Here's how the part is built. I have some questions about the finished solid (model axes, mm). A direction names the side the tool comes from. Round coordinates to 2 decimals unless told otherwise and drop trailing zeros. Loops run counter-clockwise (first coordinate to the right, second up) from the corner with the lowest first, then second, coordinate; pieces in that order, holes last. Notation, with made-up numbers: M -34,-11.5 L 20,-11.5 A9 ccw 20,-5.5 Z; hole C 73.5,19.5 d11. An arc over 180 degrees is marked long. Answer as a JSON object with one key per item and string values.
from build123d import *

# Parameters (mm, degrees)
SKETCH002_W     = 16
SKETCH002_H     = 25.5
PAD_DEPTH       = 1.5
SKETCH003_R     = 2.25
PAD001_DEPTH    = 2.9
SKETCH004_R     = 2.25
PAD002_DEPTH    = 2.9
POCKET_DEPTH    = 11.35
POCKET001_DEPTH = 11.35
FILLET_R        = 1.2


with BuildPart() as part:
    # Sketch002 → Pad (new body)
    with BuildSketch(Plane.XY):
        Rectangle(SKETCH002_W, SKETCH002_H)
        with BuildLine():
            ThreePointArc((1, 4.75), (2.5, 3.25), (4, 4.75))
            Line((4, 4.75), (4, 5.25))
            ThreePointArc((4, 5.25), (2.5, 6.75), (1, 5.25))
            Line((1, 4.75), (1, 5.25))
        make_face(mode=Mode.SUBTRACT)
        with BuildLine():
            ThreePointArc((-1, -4.75), (-2.5, -3.25), (-4, -4.75))
            Line((-4, -4.75), (-4, -5.25))
            ThreePointArc((-4, -5.25), (-2.5, -6.75), (-1, -5.25))
            Line((-1, -4.75), (-1, -5.25))
        make_face(mode=Mode.SUBTRACT)
    extrude(amount=PAD_DEPTH)

    # Sketch003 → Pad001 (join)
    with BuildSketch(Plane.XZ.offset(12.75)):
        with BuildLine():
            ThreePointArc((12.25, 0), (18.500032, 6.25), (12.25, 12.5))
            Line((12.25, 12.5), (0.660254, 12.5))
            Line((0.660254, 12.5), (-8, 7.5))
            Line((-8, 7.5), (-8, 0))
            Line((-8, 0), (12.25, 0))
        make_face()
        with Locations((12.25, 6.25)):
            Circle(SKETCH003_R, mode=Mode.SUBTRACT)
    extrude(amount=-PAD001_DEPTH)

    # Sketch004 → Pad002 (join)
    with BuildSketch(Plane.XZ.offset(-12.75)):
        with BuildLine():
            Line((12.25, 0), (-8, 0))
            Line((-8, 0), (-8, 7.5))
            Line((-8, 7.5), (0.660254, 12.5))
            Line((0.660254, 12.5), (12.25, 12.5))
            ThreePointArc((12.25, 0), (18.500035, 6.25), (12.25, 12.5))
        make_face()
        with Locations((12.250035, 6.25)):
            Circle(SKETCH004_R, mode=Mode.SUBTRACT)
    extrude(amount=PAD002_DEPTH)

    # Sketch005 → Pocket (cut)
    with BuildSketch(Plane.XZ.offset(11.35)):
        with BuildLine():
            Line((18.6, 12.5), (18.6, 0))
            Line((8, 0), (18.6, 0))
            Line((8, 1.005956), (8, 0))
            ThreePointArc((6.50892, 9.8), (5.594985, 5.121605), (8, 1.005956))
            Line((6.50892, 9.8), (11.5, 9.8))
            Line((11.5, 9.8), (11.5, 12.5))
            Line((11.5, 12.5), (18.6, 12.5))
        make_face()
    extrude(amount=-POCKET_DEPTH, mode=Mode.SUBTRACT)

    # Sketch006 → Pocket001 (cut)
    with BuildSketch(Plane.XZ.offset(-11.35)):
        with BuildLine():
            Line((18.6, 12.5), (18.6, 0))
            Line((8, 0), (18.6, 0))
            Line((8, 1.005956), (8, 0))
            ThreePointArc((6.50892, 9.8), (5.594985, 5.121605), (8, 1.005956))
            Line((6.50892, 9.8), (11.5, 9.8))
            Line((11.5, 9.8), (11.5, 12.5))
            Line((11.5, 12.5), (18.6, 12.5))
        make_face()
    extrude(amount=POCKET001_DEPTH, mode=Mode.SUBTRACT)

    # Fillet
    fillet_edges = [part.edges().sort_by_distance(p)[0] for p in [
        (-0.272916, 9.85, 1.5),
        (-0.272916, -9.85, 1.5),
    ]]
    fillet(fillet_edges, radius=FILLET_R)


solid = part.part
Item 1: I want a section at C-C on y = 10.5. List the corners of the cut face in (x, z) for me, plus the area to 3 significant figures.
Solution:
{"outline": "M -8,0 L 8,0 L 8,1.01 A6.75 cw 6.51,9.8 L 11.5,9.8 L 11.5,12.5 L 0.66,12.5 L -8,7.5 Z", "area": "171 mm2"}
Item 2: We'd pull the mould along Y, two halves only. Please class faces 6 (the face through (5, 12.75, 6)), 7 (the face through (10, -12.1, 6.3)), 8 (the face through (2.47, 3.25, 0.74)): +Y half, -Y half, draft (parallel to the pull), parting line (faces both ways), or undercut.
Solution:
{"face 6": "+Y half", "face 7": "draft", "face 8": "undercut"}
Item 3: If I drill on L1, parallel to Y at x = 13, z = 9; L2, parallel to Y at x = -6, z = 8.25; L3, parallel to Z at x = 12.25, y = -11.65, over which ranges is the centre line in solid material (lowest first)? Write a range as from..to.
Solution:
{"L1": "y = -12.75..-11.35, 11.35..12.75", "L2": "y = -12.75..-9.85, 9.85..12.75", "L3": "z = 0..4, 8.5..12.5"}
Item 4: I want a section at D-D on x = 13.25. List the corners of the cut face in (y, z) for me.
Solution:
{"outline": "M -12.75,0.08 L -11.35,0.08 L -11.35,4.23 L -12.75,4.23 Z; M -12.75,8.27 L -11.35,8.27 L -11.35,12.42 L -12.75,12.42 Z; M 11.35,0.08 L 12.75,0.08 L 12.75,4.23 L 11.35,4.23 Z; M 11.35,8.27 L 12.75,8.27 L 12.75,12.42 L 11.35,12.42 Z"}
Item 5: I want a section at A-A on x = 2.5. List the corners of the cut face in (y, z) for me, plus the area to 3 significant figures.
Solution:
{"outline": "M -12.75,0 L 3.25,0 L 3.25,1.5 L -8.65,1.5 A1.2 cw -9.85,2.7 L -9.85,12.5 L -12.75,12.5 Z; M 6.75,0 L 12.75,0 L 12.75,12.5 L 9.85,12.5 L 9.85,2.7 A1.2 cw 8.65,1.5 L 6.75,1.5 Z", "area": "97.4 mm2"}
Item 6: I want a section at B-B on z = 7. List the corners of the cut face in (x, y) for me, plus the area to 3 significant figures.
Solution:
{"outline": "M -8,-12.75 L 10.13,-12.75 L 10.13,-11.35 L 5.54,-11.35 L 5.54,-9.85 L -8,-9.85 Z; M -8,9.85 L 5.54,9.85 L 5.54,11.35 L 10.13,11.35 L 10.13,12.75 L -8,12.75 Z; M 14.37,-12.75 L 18.45,-12.75 L 18.45,-11.35 L 14.37,-11.35 Z; M 14.37,11.35 L 18.45,11.35 L 18.45,12.75 L 14.37,12.75 Z", "area": "103 mm2"}
Item 7: For P1, Ø2, axis at y = -7.5, z = 5.5, coming from the -X side; P2, Ø2, axis at x = 4, y = 1, coming from the +Z side; P3, Ø12.5, axis at x = -3.5, y = 3, coming from the +Z side; P4, Ø1.2, axis at y = -10.5, z = 11.5, coming from the +X side, each with a flat end and sliding along its axis, tell me the tip position at first contact or that it passes through.
Solution:
{"P1": "passes through", "P2": "stops at z = 1.5", "P3": "stops at z = 1.66", "P4": "stops at x = 11.5"}
Item 8: For faces 1 (the face through (-0.381, 9.489, 1.842)), 2 (the face through (8, -0.2, 0.5)), 3 (the face through (-2.53, -6.75, 0.74)), 4 (the face through (11.5, -11, 11)), 5 (the face through (7.577, -0.053, 1.379)), which set-ups out of +Z, -Z, +X, -X, +Y, -Y let a thin tool reach every point of the face, with its end or its side?
Solution:
{"face 1": "+Z, +X, -X", "face 2": "-Z, +X", "face 3": "+Z, -Z", "face 4": "+Z, -Z, +X", "face 5": "+X"}
